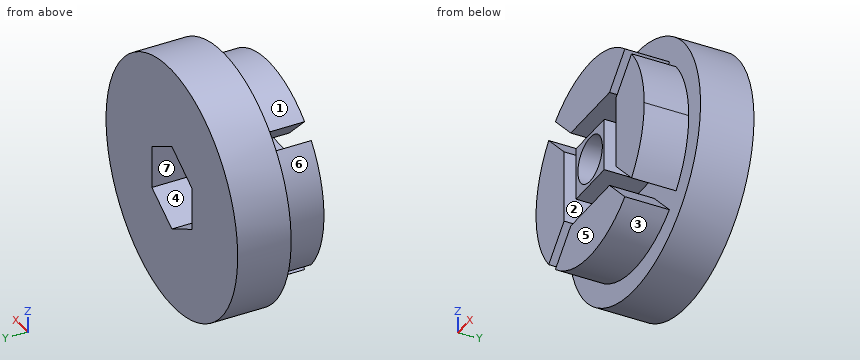
```python
from build123d import *

# Parameters (mm, degrees)
SKETCH3_W           = 6
SKETCH3_H           = 6
SKETCH3_R           = 2.6
BASE_DEPTH          = 5
BLOC_START          = 6
SKETCH8_R           = 14
SKETCH8_R_2         = 2.6
BLOC_DEPTH          = 6
NUT_PLACE_DEPTH     = 4
REINFORCEMENT_DEPTH = 5


with BuildPart() as part:
    # Sketch3 → Base (new body)
    with BuildSketch(Plane(origin=(0, 0, 0), x_dir=(1, 0, 0), z_dir=(0, 1, 0))):
        Rectangle(SKETCH3_W, SKETCH3_H)
        with Locations(Location((0, 0, 0), (0, 0, 270))):
            Circle(SKETCH3_R, mode=Mode.SUBTRACT)
    extrude(amount=-BASE_DEPTH)

    # Sketch8 → Bloc (add)
    with BuildSketch(Plane(origin=(0, 0, 0), x_dir=(1, 0, 0), z_dir=(0, 1, 0)).offset(BLOC_START)):
        with Locations(Location((0, 0, 0), (0, 0, 270))):
            Circle(SKETCH8_R)
        with Locations(Location((0, 0, 0), (0, 0, 270))):
            Circle(SKETCH8_R_2, mode=Mode.SUBTRACT)
    extrude(amount=-BLOC_DEPTH)

    # Sketch4 → Nut_place (cut)
    with BuildSketch(Plane(origin=(0, 6, 0), x_dir=(1, 0, 0), z_dir=(0, 1, 0))):
        Polygon((0, 4.907477288), (-4.25, 2.453738644), (-4.25, -2.453738644), (0, -4.907477288), (4.25, -2.453738644), (4.25, 2.453738644), align=None)
    extrude(amount=-NUT_PLACE_DEPTH, mode=Mode.SUBTRACT)

    # Sketch9 → Reinforcement (add)
    with BuildSketch(Plane.XZ):
        with BuildLine():
            ThreePointArc((11.5, 0), (10.806071801, 3.934312168), (8.808032654, 7.393819092))
            Line((8.808032654, 7.393819092), (5.539213562, 4.125))
            Line((5.539213562, 4.125), (5.539213562, -4.125))
            Line((5.539213562, -4.125), (8.808032654, -7.393819092))
            ThreePointArc((8.808032654, -7.393819092), (10.806071801, -3.934312168), (11.5, 0))
        make_face()
        with BuildLine():
            Line((-4.125, -5.539213562), (-7.393819092, -8.808032654))
            ThreePointArc((-7.393819092, -8.808032654), (0, -11.5), (7.393819092, -8.808032654))
            Line((7.393819092, -8.808032654), (4.125, -5.539213562))
            Line((4.125, -5.539213562), (-4.125, -5.539213562))
        make_face()
        with BuildLine():
            Line((-5.539213562, -4.125), (-5.539213562, 4.125))
            Line((-5.539213562, 4.125), (-8.808032654, 7.393819092))
            ThreePointArc((-8.808032654, 7.393819092), (-11.5, 0), (-8.808032654, -7.393819092))
            Line((-8.808032654, -7.393819092), (-5.539213562, -4.125))
        make_face()
        with BuildLine():
            ThreePointArc((7.393819092, 8.808032654), (0, 11.5), (-7.393819092, 8.808032654))
            Line((-7.393819092, 8.808032654), (-4.125, 5.539213562))
            Line((-4.125, 5.539213562), (4.125, 5.539213562))
            Line((4.125, 5.539213562), (7.393819092, 8.808032654))
        make_face()
    extrude(amount=REINFORCEMENT_DEPTH)


solid = part.part
```
Can you work these out from the model? Positions are in its coordinate system, mm. Face numbers are marked on the shaded views. A direction names the side the tool comes from. Round coordinates to 2 decimals unless told otherwise and drop trailing zeros. Loops run counter-clockwise (first coordinate to the right, second up) from the corner with the lowest first, then second, coordinate; pieces in that order, holes last. Notation, with made-up numbers: (-28, -12) -> (24, -12) arc R23 ccw to (24, 22) -> close; hole circle Ø7 at (48.25, 61). An arc over 180 degrees is marked (long way). One line per item, written item: value. Start each with the question number.
1. If I drill on probe 1 along X at (y, z) = (-3, 0); probe 2 along Y at (x, z) = (-2, 4.75); probe 3 along Z at (x, y) = (-0.25, -0.5), over which ranges is the centre line in solid material (lowest first)?
2. If we section it at A-A, the plane y = -1.75: Write out the boundary of the cut face in (x, z) (3 decimals), then the cut area to 3 significant figures.
3. If we mould it in two halves opening along Z, with no side actions, what happens to the marked faces 5, 6 and 7? For each: pulls with the +Z half, pulls with the -Z half, needs draft (parallel to the pull), parting line crosses it, or undercut.
4. If we section it at D-D, the plane z = 9.5: Write out the boundary of the cut face in (x, y), then the cut area to 3 significant figures.
5. For the marked faces 1, 2, 3 and 4, which set-ups out of +Z, -Z, +X, -X, +Y, -Y let a thin tool reach every point of the face, with its end or its side?
6. If we section it at B-B, the plane y = 2.75: Write out the boundary of the cut face in (x, z), then the cut area to 3 significant figures.
7. For pin 1 (2.5 mm diameter, centred on y = -1.5, z = 1.5, fed in from -X); pin 2 (2.5 mm diameter, centred on x = -1, y = -1.5, fed in from -Z); pin 3 (2.5 mm diameter, centred on x = 1.5, y = -3.5, fed in from +Z), each with a flat end and sliding along its axis, tell me the tip position at first contact or that it passes through.
8. If we section it at C-C, the plane x = 1: Write out the boundary of the cut face in (y, z).
Calculated:
1. probe 1: x = -11.5 to -5.54, -3 to -2.6, 2.6 to 3, 5.54 to 11.5
1. probe 2: y = 0 to 6
1. probe 3: z = -11.5 to -5.54, -3 to -2.59, 2.59 to 3, 5.54 to 11.5
2. outline: (-8.808, -7.394) -> (-5.539, -4.125) -> (-5.539, 4.125) -> (-8.808, 7.394) arc R11.5 ccw to start; (-7.394, -8.808) arc R11.5 ccw to (7.394, -8.808) -> (4.125, -5.539) -> (-4.125, -5.539) -> close; (-7.394, 8.808) -> (-4.125, 5.539) -> (4.125, 5.539) -> (7.394, 8.808) arc R11.5 ccw to start; (-3, -3) -> (3, -3) -> (3, 3) -> (-3, 3) -> close; (5.539, -4.125) -> (8.808, -7.394) arc R11.5 ccw to (8.808, 7.394) -> (5.539, 4.125) -> close; hole circle Ø5.2 at (0, 0)
2. area: 274 mm²
3. face 5: needs draft
3. face 6: parting line crosses it
3. face 7: undercut
4. outline: (-10.28, 0) -> (-6.48, 0) -> (-6.48, -5) -> (6.48, -5) -> (6.48, 0) -> (10.28, 0) -> (10.28, 6) -> (-10.28, 6) -> close
4. area: 188 mm²
5. face 1: +Z, -Y
5. face 2: -Y
5. face 3: -Z, -Y
5. face 4: +Y
6. outline: circle Ø28 at (0, 0); hole (-4.25, -2.45) -> (0, -4.91) -> (4.25, -2.45) -> (4.25, 2.45) -> (0, 4.91) -> (-4.25, 2.45) -> close
6. area: 553 mm²
7. pin 1: stops at x = -11.5
7. pin 2: stops at z = -11.5
7. pin 3: stops at z = 11.5
8. outline: (-5, -11.46) -> (0, -11.46) -> (0, -13.96) -> (6, -13.96) -> (6, -4.33) -> (2, -4.33) -> (2, -2.4) -> (-5, -2.4) -> (-5, -3) -> (0, -3) -> (0, -5.54) -> (-5, -5.54) -> close; (-5, 2.4) -> (2, 2.4) -> (2, 4.33) -> (6, 4.33) -> (6, 13.96) -> (0, 13.96) -> (0, 11.46) -> (-5, 11.46) -> (-5, 5.54) -> (0, 5.54) -> (0, 3) -> (-5, 3) -> close
